Source: CAD feature listing. Evaluate the final solid. Frame: model axes, mm. Face numbers are marked on the shaded views. Give positions to 0.01 mm unless a question says otherwise; leave off trailing zeros. Order: outer loops, then holes, each group sorted by start corner. A loop starts at its lowest first (then second) coordinate and runs counter-clockwise, first axis right, second up. Notation, with made-up numbers: (-32.75, 81) -> (-16.75, 81) arc R26 ccw to (-16.75, 109) -> close; hole circle Ø8 at (-11.5, 14.25). An arc over 180 degrees is marked (long way). Answer in a Markdown table with one row per item.
```python
from build123d import *


with BuildPart() as part:
    # Эскиз1 → Повернуть1 (revolve)
    with BuildSketch(Plane.XY):
        with BuildLine():
            Line((0.970205183, 19.32988738), (0, 19.139))
            Line((0, 19.139), (0, 22.9))
            ThreePointArc((0, 22.9), (0.175735931, 23.324264069), (0.6, 23.5))
            Line((0.6, 23.5), (13.4, 23.5))
            ThreePointArc((13.4, 23.5), (13.824264069, 23.324264069), (14, 22.9))
            Line((14, 22.9), (14, 21.893492934))
            Line((14, 21.893492934), (13.012426118, 21.699188271))
            Line((13.012426118, 21.699188271), (14, 16.578811729))
            Line((14, 16.578811729), (14, 17.178811729))
            Line((14, 17.178811729), (16.4, 17.178811729))
            ThreePointArc((16.4, 17.178811729), (16.824264069, 17.003075798), (17, 16.578811729))
            Line((17, 16.578811729), (17, 13.1))
            ThreePointArc((17, 13.1), (16.824264069, 12.675735931), (16.4, 12.5))
            Line((16.4, 12.5), (0.6, 12.5))
            ThreePointArc((0.6, 12.5), (0.175735931, 12.675735931), (0, 13.1))
            Line((0, 13.1), (0, 14.299564132))
            Line((0, 14.299564132), (1.940410366, 14.299564132))
            Line((1.940410366, 14.299564132), (0.970205183, 19.32988738))
        make_face()
    revolve(axis=Axis((-882.527700014, 0, 0), (1, 0, 0)))


solid = part.part
```
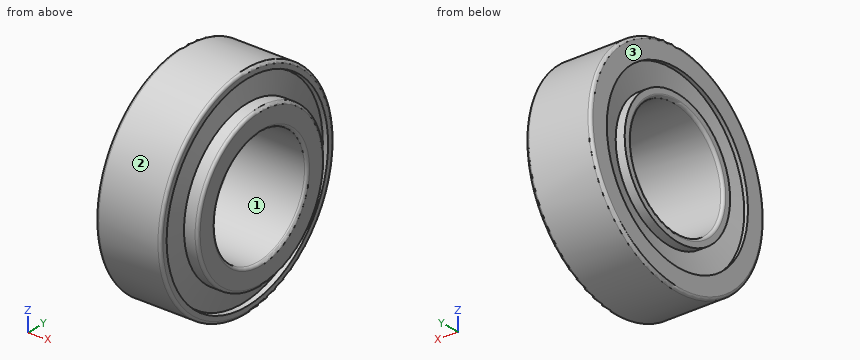
(1) Pull-direction query (Y, two-part tool) for the marked faces 1, 2 and 3; classes: +Y half, -Y half, draft (parallel to the pull), parting line (faces both ways), or undercut.
A:
| item | result |
|---|---|
| face 1 | undercut |
| face 2 | parting line |
| face 3 | draft |
(2) Section query A-A (x = 9.75). Return the cut outline in (y, z).
A:
| item | result |
|---|---|
| outline | circle Ø47 at (0, 0); hole circle Ø25 at (0, 0) |
(3) First-contact query: pin 1 Ø4 at (x, z) = (8.5, -15.5) entering from -Y; pin 2 Ø3 at (x, y) = (9.5, 16) entering from -Z; pin 3 Ø10 at (x, y) = (2.5, 7) entering from -Z. Flat tips, straight axial feed; report the tip coordinate or a pass-through.
A:
| item | result |
|---|---|
| pin 1 | stops at y = -19.24 |
| pin 2 | stops at z = -18.49 |
| pin 3 | stops at z = -23.41 |
(4) Ray query, probe 1 along Z at (x, y) = (5.5, 0); probe 2 along X at (y, z) = (16, 16); probe 3 along Z at (x, y) = (10, 2). Return the intervals inside material, ascending.
A:
| item | result |
|---|---|
| probe 1 | z = -23.5 to -12.5, 12.5 to 23.5 |
| probe 2 | x = 0 to 14 |
| probe 3 | z = -23.41 to -12.34, 12.34 to 23.41 |
